Can you work these out from the model? Positions are in its coordinate system, mm. Face numbers are marked on the shaded views. A direction names the side the tool comes from. Give positions to 0.01 mm unless a question says otherwise; leave off trailing zeros. Write each loop counter-clockwise with the first axis right and the second up, starting at its lowest first coordinate (ties: lowest second). Pieces come first, ordered by that corner, then holes.
1. If I drill on probe 1 along Y at (x, z) = (-0.5, 2.9) (3 decimals); probe 2 along Y at (x, z) = (-9, 2.75); probe 3 along X at (y, z) = (-14.5, 0.4), over which ranges is the centre line in solid material (lowest first)?
2. Suppose I cut it at B-B (x = -17). Please give me the cut outline in (y, z).
3. I'm going to push a flat-ended pin straight in: pin 1 (1 mm diameter, centred on y = 16.5, z = 3, fed in from +X). Where does the tip first touch, or does it pass through?
4. On a 3-axis mill with a long thin cutter (end or side, diameter ignored), from which of +Z, -Z, +X, -X, +Y, -Y can I reach the whole of each face in a straight line? I mean the marked faces 4 and 5. Say none if no direction works.
5. Thinking about a two-plate mould opening in X: for the marked faces 1, 2 and 3, which applies, pulls with the +X half, pulls with the -X half, needs draft (parallel to the pull), parting line crosses it, or undercut?
6. Suppose I cut it at A-A (z = 0.7). Give the number of separate pieces and of enclosed holes in the cut face, and give its area (3 significant figures).
```python
from build123d import *

# Parameters (mm, degrees)
SKETCH_R        = 25
PAD_DEPTH       = 4
POCKET_DEPTH    = 5
POCKET001_DEPTH = 5


with BuildPart() as part:
    # Sketch → Pad (new body)
    with BuildSketch(Plane.XY):
        Circle(SKETCH_R)
    extrude(amount=PAD_DEPTH)

    # Sketch003 → Pocket (cut)
    with BuildSketch(Plane(origin=(0, 0, 0), x_dir=(-1, 0, 0), z_dir=(0, 0, 1))):
        with BuildLine():
            ThreePointArc((-10, 0), (-12.5, 2.357995), (-15, 0))
            add(Edge.make_bspline(
                [(-15, 0), (-15.375, -2.945243), (-15.089089, -6.058788), (-14.076175, -9.167592), (-12.324531, -12.071008), (-9.890344, -14.561821), (-6.900284, -16.456905), (-3.534292, -17.625), (0, -18)],
                knots=[0, 0, 0, 0, 0, 0, 0, 0, 0, 1.862096, 1.862096, 1.862096, 1.862096, 1.862096, 1.862096, 1.862096, 1.862096, 1.862096], degree=8))
            ThreePointArc((0, -18), (1.91492, -15.5), (0, -13))
            add(Edge.make_bspline(
                [(-10, 0), (-10.375, -1.963495), (-10.309393, -4.095292), (-9.737085, -6.280026), (-8.628237, -8.374714), (-7.002778, -10.222731), (-4.936788, -11.677209), (-2.552544, -12.625), (0, -13)],
                knots=[0, 0, 0, 0, 0, 0, 0, 0, 0, 1.862096, 1.862096, 1.862096, 1.862096, 1.862096, 1.862096, 1.862096, 1.862096, 1.862096], degree=8))
        make_face()
    extrude(amount=POCKET_DEPTH, mode=Mode.SUBTRACT)

    # Sketch005 → Pocket001 (cut)
    with BuildSketch(Plane(origin=(0, 0, 0), x_dir=(-1, 0, 0), z_dir=(0, 0, 1))):
        with BuildLine():
            ThreePointArc((10, 0), (12.5, -2.707209), (15, 0))
            add(Edge.make_bspline(
                [(15, 0), (15.375, 2.945243), (15.089089, 6.058788), (14.076175, 9.167592), (12.324531, 12.071008), (9.890344, 14.561821), (6.900284, 16.456905), (3.534292, 17.625), (0, 18)],
                knots=[0, 0, 0, 0, 0, 0, 0, 0, 0, 1.862096, 1.862096, 1.862096, 1.862096, 1.862096, 1.862096, 1.862096, 1.862096, 1.862096], degree=8))
            ThreePointArc((0, 18), (-2.555164, 15.5), (0, 13))
            add(Edge.make_bspline(
                [(10, 0), (10.375, 1.963495), (10.309393, 4.095292), (9.737085, 6.280026), (8.628237, 8.374714), (7.002778, 10.222731), (4.936788, 11.677209), (2.552544, 12.625), (0, 13)],
                knots=[0, 0, 0, 0, 0, 0, 0, 0, 0, 1.862096, 1.862096, 1.862096, 1.862096, 1.862096, 1.862096, 1.862096, 1.862096, 1.862096], degree=8))
        make_face()
    extrude(amount=POCKET001_DEPTH, mode=Mode.SUBTRACT)


solid = part.part
```
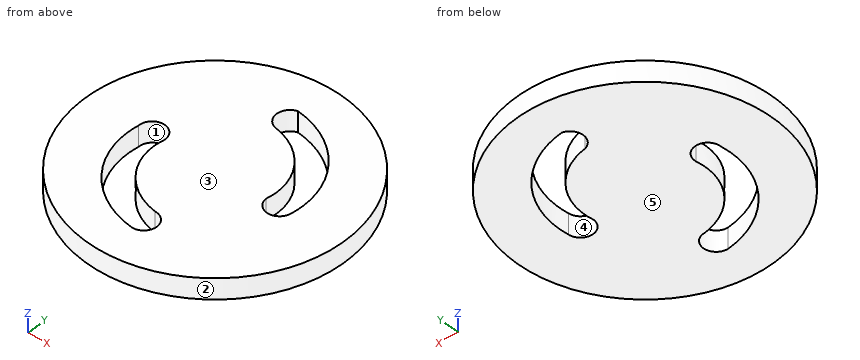
Checks:
1. probe 1: y = -24.995 to -17.94, -12.916 to 13.192, 17.808 to 24.995
1. probe 2: y = -23.32 to -14.34, -6.7 to 23.32
1. probe 3: x = -20.37 to -8.79, 2.35 to 20.37
2. outline: (-18.33, 0) - (18.33, 0) - (18.33, 4) - (-18.33, 4) - close
3. pin 1: stops at x = 19.21
4. face 4: +Z, -Z
4. face 5: -Z, +X, -X, +Y, -Y
5. face 1: undercut
5. face 2: parting line crosses it
5. face 3: needs draft
6. separate pieces: 1
6. enclosed holes: 2
6. area: 1,710 mm2
